Geometry: final body of the model. Coordinates: model frame, mm. A direction names the side the tool comes from. Round coordinates to 2 decimals unless told otherwise and drop trailing zeros. Loops run counter-clockwise (first coordinate to the right, second up) from the corner with the lowest first, then second, coordinate; pieces in that order, holes last. Notation, with made-up numbers: (70.25, -33) -> (77.25, -33) arc R35 ccw to (77.25, 6) -> close; hole circle Ø5 at (-5, 10.25). An arc over 180 degrees is marked (long way). Answer in a Markdown table with one row per item.
```python
from build123d import *

# Parameters (mm, degrees)
SKETCH3_R           = 11
SKETCH3_R_2         = 3.98
BOSS_EXTRUDE1_DEPTH = 3.48
SKETCH4_R           = 9.8
SKETCH4_R_2         = 5.68
CUT_EXTRUDE1_DEPTH  = 0.2


with BuildPart() as part:
    # Sketch3 → Boss-Extrude1 (new, symmetric)
    with BuildSketch(Plane(origin=(0, 0, 0), x_dir=(1, 0, 0), z_dir=(0, 1, 0))):
        with Locations(Location((0, 0, 0), (0, 0, 270))):
            Circle(SKETCH3_R)
        with Locations(Location((0, 0, 0), (0, 0, 270))):
            Circle(SKETCH3_R_2, mode=Mode.SUBTRACT)
    extrude(amount=BOSS_EXTRUDE1_DEPTH, both=True)

    # Sketch4 → Cut-Extrude1 (cut)
    with BuildSketch(Plane(origin=(0, 3.48, 0), x_dir=(1, 0, 0), z_dir=(0, 1, 0))):
        with Locations(Location((0, 0, 0), (0, 0, 270))):
            Circle(SKETCH4_R)
        with Locations(Location((0, 0, 0), (0, 0, 270))):
            Circle(SKETCH4_R_2, mode=Mode.SUBTRACT)
    cut_extrude1 = extrude(amount=-CUT_EXTRUDE1_DEPTH, mode=Mode.SUBTRACT)

    # Mirror1: Cut-Extrude1 across plane
    add(cut_extrude1.mirror(Plane.ZX), mode=Mode.SUBTRACT)


solid = part.part
```
Item 1: Section query B-B, the plane z = 0. Output: boundary loops of the cut face in (x, y), and give its area (3 significant figures).
Ans:
| item | result |
|---|---|
| outline | (-11, -3.48) -> (-9.8, -3.48) -> (-9.8, -3.28) -> (-5.68, -3.28) -> (-5.68, -3.48) -> (-3.98, -3.48) -> (-3.98, 3.48) -> (-5.68, 3.48) -> (-5.68, 3.28) -> (-9.8, 3.28) -> (-9.8, 3.48) -> (-11, 3.48) -> close; (3.98, -3.48) -> (5.68, -3.48) -> (5.68, -3.28) -> (9.8, -3.28) -> (9.8, -3.48) -> (11, -3.48) -> (11, 3.48) -> (9.8, 3.48) -> (9.8, 3.28) -> (5.68, 3.28) -> (5.68, 3.48) -> (3.98, 3.48) -> close |
| area | 94.4 mm2 |
Item 2: Section query C-C, the plane y = 1.25. Output: boundary loops of the cut face in (x, z), and give its area (3 significant figures).
Ans:
| item | result |
|---|---|
| outline | circle Ø22 at (0, 0); hole circle Ø7.96 at (0, 0) |
| area | 330 mm2 |
Item 3: Section query D-D, the plane x = 8.75. Output: boundary loops of the cut face in (y, z), and give its area (3 significant figures).
Ans:
| item | result |
|---|---|
| outline | (-3.48, -6.67) -> (3.48, -6.67) -> (3.48, -4.41) -> (3.28, -4.41) -> (3.28, 4.41) -> (3.48, 4.41) -> (3.48, 6.67) -> (-3.48, 6.67) -> (-3.48, 4.41) -> (-3.28, 4.41) -> (-3.28, -4.41) -> (-3.48, -4.41) -> close |
| area | 89.3 mm2 |
Item 4: Section query A-A, the plane x = 0. Output: boundary loops of the cut face in (y, z), and give its area (3 significant figures).
Ans:
| item | result |
|---|---|
| outline | (-3.48, -11) -> (3.48, -11) -> (3.48, -9.8) -> (3.28, -9.8) -> (3.28, -5.68) -> (3.48, -5.68) -> (3.48, -3.98) -> (-3.48, -3.98) -> (-3.48, -5.68) -> (-3.28, -5.68) -> (-3.28, -9.8) -> (-3.48, -9.8) -> close; (-3.48, 3.98) -> (3.48, 3.98) -> (3.48, 5.68) -> (3.28, 5.68) -> (3.28, 9.8) -> (3.48, 9.8) -> (3.48, 11) -> (-3.48, 11) -> (-3.48, 9.8) -> (-3.28, 9.8) -> (-3.28, 5.68) -> (-3.48, 5.68) -> close |
| area | 94.4 mm2 |
Item 5: Ray query, L1, parallel to X at y = 1.75, z = 0; L2, parallel to Y at x = 1.75, z = 8; L3, parallel to Z at x = 2.25, y = 0.75. Return the intervals inside material, ascending.
Ans:
| item | result |
|---|---|
| L1 | -11 to -3.98, 3.98 to 11 |
| L2 | -3.28 to 3.28 |
| L3 | -10.77 to -3.28, 3.28 to 10.77 |
Item 6: Mould query, pull axis Z, two halves, no side actions, for faces 3 (the cylindrical face through (-10.74, 0.05, -2.38)), 4 (the flat face through (-4, -3.48, 2)), 5 (the cylindrical face through (3.946, -0.049, -0.518)), 6 (the flat face through (-4.2, -3.28, 4.2)). Classes: released by +Z, released by -Z, zero draft, split by the parting line, or undercut.
Ans:
| item | result |
|---|---|
| face 3 | split by the parting line |
| face 4 | zero draft |
| face 5 | undercut |
| face 6 | undercut |
Item 7: Set-up query: faces 1 (the flat face through (-4.2, 3.28, 4.2)), 2 (the flat face through (-1, 3.48, -10)). Return all of +Z, -Z, +X, -X, +Y, -Y with unobstructed straight access to the full face (end or side cutting, diameter ignored); none if empty.
Ans:
| item | result |
|---|---|
| face 1 | +Y |
| face 2 | +Z, -Z, +X, -X, +Y |
